from build123d import *

# Parameters (mm, degrees)
RESSALTO_EXTRUS_O1_DEPTH                = 10
ESBO_O2_R                               = 5.25
CORTE_EXTRUS_O1_DEPTH                   = 16
CORTE_EXTRUS_O1_DEPTH_BACK              = 31.8
CBORE_FOR_M5_HEX_HEAD_BOLT1_D           = 3.2
CBORE_FOR_M5_HEX_HEAD_BOLT1_CBORE_D     = 6
CBORE_FOR_M5_HEX_HEAD_BOLT1_CBORE_DEPTH = 16.5
M3_CLEARANCE_HOLE5_D                    = 3.2


with BuildPart() as part:
    # Esboço1 → Ressalto-extrusão1 (new body)
    with BuildSketch(Plane.XY):
        with BuildLine():
            Line((115.646593224, -302.7659332), (115.646593224, -295.7159332))
            Line((115.646593224, -295.7159332), (91.646593224, -295.7159332))
            Line((91.646593224, -295.7159332), (91.646593224, -302.7659332))
            ThreePointArc((91.646593224, -302.7659332), (103.646593224, -314.7659332), (115.646593224, -302.7659332))
        make_face()
    extrude(amount=RESSALTO_EXTRUS_O1_DEPTH)

    # Esboço2 → Corte-extrusão1 (cut, two sides)
    with BuildSketch(Plane.XY.offset(10)) as corte_extrus_o1_sk:
        with Locations((103.646593224, -302.7659332)):
            Circle(ESBO_O2_R)
    extrude(amount=CORTE_EXTRUS_O1_DEPTH, mode=Mode.SUBTRACT)
    extrude(corte_extrus_o1_sk.sketch, amount=-CORTE_EXTRUS_O1_DEPTH_BACK, mode=Mode.SUBTRACT)

    # CBORE for M5 Hex Head Bolt1 (through all)
    with Locations(Plane(origin=(0, -314.7159332, 0), x_dir=(-1, 0, 0), z_dir=(0, -1, 0))):
        with Locations((-95.596593224, -5.949346208), (-110.596593224, -5.949346208)):
            CounterBoreHole(CBORE_FOR_M5_HEX_HEAD_BOLT1_D / 2, CBORE_FOR_M5_HEX_HEAD_BOLT1_CBORE_D / 2, CBORE_FOR_M5_HEX_HEAD_BOLT1_CBORE_DEPTH)

    # M3 Clearance Hole5 (through all)
    with Locations(Plane.XY.offset(10)):
        with Locations((95.681870132, -302.765933199), (103.646593224, -310.730656291), (111.611316315, -302.765933199)):
            Hole(M3_CLEARANCE_HOLE5_D / 2)


solid = part.part
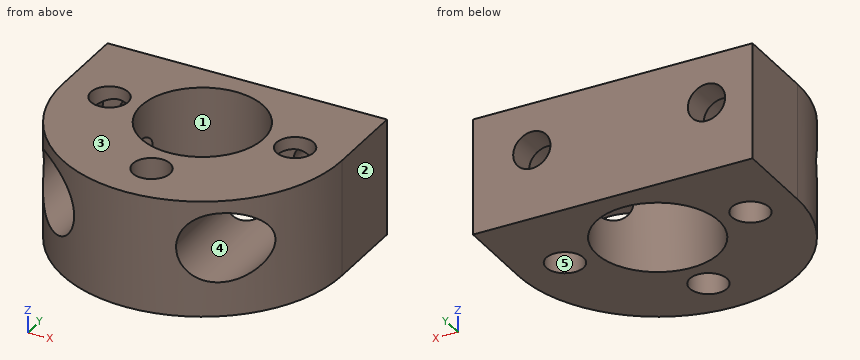
Can you work these out from the model? Positions are in its coordinate system, mm. Face numbers are marked on the shaded views. A direction names the side the tool comes from. Coordinates: 2 decimals unless noted, no trailing zeros. Loops run counter-clockwise (first coordinate to the right, second up) from the corner with the lowest first, then second, coordinate; pieces in that order, holes last. Notation, with made-up numbers: M 59,81 L 94,81 A30 ccw 94,104 Z; hole C 33,12 d3. An arc over 180 degrees is marked long. Return JSON: item names as keys, results as strings. Group by question number.
Item 1: Imagine slicing it at C-C (x = 102.5). Please give me the cut outline in (y, z), and give its area (3 significant figures).
Item 2: Imagine slicing it at D-D (y = -303.5). Please give me the cut outline in (x, z).
Item 3: Thinking about a two-plate mould opening in X: for the marked faces 1, 2 and 3, which applies, released by +X, released by -X, zero draft, split by the parting line, or undercut?
Item 4: Imagine slicing it at A-A (z = 6.5). Please give me the cut outline in (x, y).
Item 5: Imagine slicing it at B-B (y = -300.5). Please give me the cut outline in (x, z), and give its area (3 significant figures).
Item 6: I'm going to push flat-ended pins straight in: pin 1 Ø2.5 at (x, z) = (95.6, 5.95) entering from -Y; pin 2 Ø6 at (y, z) = (-306, 1) entering from +X; pin 3 Ø6 at (x, y) = (107, -304) entering from -Z; pin 4 Ø2 at (y, z) = (-312.5, 2.5) entering from -X. Where does each tip first touch, or does it pass through?
Item 7: On a 3-axis mill with a long thin cutter (end or side, diameter ignored), from which of +Z, -Z, +X, -X, +Y, -Y can I reach the whole of each face in a straight line? I mean the marked faces 4 and 5. Say none if no direction works.
Item 8: If I drill on L1, parallel to X at y = -302.5, z = 1; L2, parallel to X at y = -304, z = 3.75; L3, parallel to X at y = -301.75, z = 8.25, over which ranges is the centre line in solid material (lowest first)? Write a range as from..to.
Verdict:
{
 "1": {"outline": "M -314.71,0 L -311.85,0 L -311.85,10 L -314.71,10 Z; M -309.61,0 L -307.89,0 L -307.89,10 L -309.61,10 Z; M -297.64,0 L -295.72,0 L -295.72,10 L -297.64,10 Z", "area": "65.2 mm^2"},
 "2": {"outline": "M 91.67,0 L 94.26,0 L 94.26,3.26 A3 cw 94.26,8.64 L 94.26,10 L 91.67,10 Z; M 97.1,0 L 98.45,0 L 98.45,5.02 A3 cw 97.1,3.36 Z; M 97.1,8.54 A3 cw 98.45,6.88 L 98.45,10 L 97.1,10 Z; M 108.85,0 L 110.19,0 L 110.19,2.98 A3 cw 108.85,3.51 Z; M 108.85,8.38 A3 cw 110.19,8.92 L 110.19,10 L 108.85,10 Z; M 113.03,0 L 115.62,0 L 115.62,10 L 113.03,10 L 113.03,7.7 A3 cw 113.03,4.2 Z"},
 "3": {"face 1": "undercut", "face 2": "released by +X", "face 3": "zero draft"},
 "4": {"outline": "M 91.65,-302.77 A12 ccw 92.65,-307.56 L 92.65,-298.22 L 94.09,-298.22 L 94.09,-295.72 L 91.65,-295.72 Z; M 97.1,-298.22 L 98.55,-298.22 L 98.55,-301.52 A5.25 cw 107.65,-299.37 L 107.65,-298.22 L 109.09,-298.22 L 109.09,-295.72 L 97.1,-295.72 Z; M 98.55,-313.63 A12 ccw 107.65,-314.08 L 107.65,-306.17 A5.25 cw 98.55,-304.01 Z; M 112.1,-298.22 L 113.55,-298.22 L 113.55,-309.55 A12 ccw 115.65,-302.77 L 115.65,-295.72 L 112.1,-295.72 Z; hole C 103.65,-310.73 d3.2"},
 "5": {"outline": "M 91.65,0 L 98.91,0 L 98.91,10 L 91.65,10 Z; M 108.38,0 L 115.65,0 L 115.65,10 L 108.38,10 L 108.38,7.97 A3 cw long 108.38,3.93 Z; hole C 95.6,5.95 d6", "area": "90.9 mm^2"},
 "6": {"pin 1": "passes through", "pin 2": "stops at x = 115.64", "pin 3": "stops at z = 0", "pin 4": "stops at x = 95.42"},
 "7": {"face 4": "-Y", "face 5": "+Z, -Z"},
 "8": {"L1": "x = 91.65..94.1, 97.26..98.4, 108.89..110.03, 113.19..115.65", "L2": "x = 91.71..93.56, 97.64..98.54, 112.64..115.58", "L3": "x = 91.65..93.67, 97.52..98.5, 112.85..115.65"}
}
